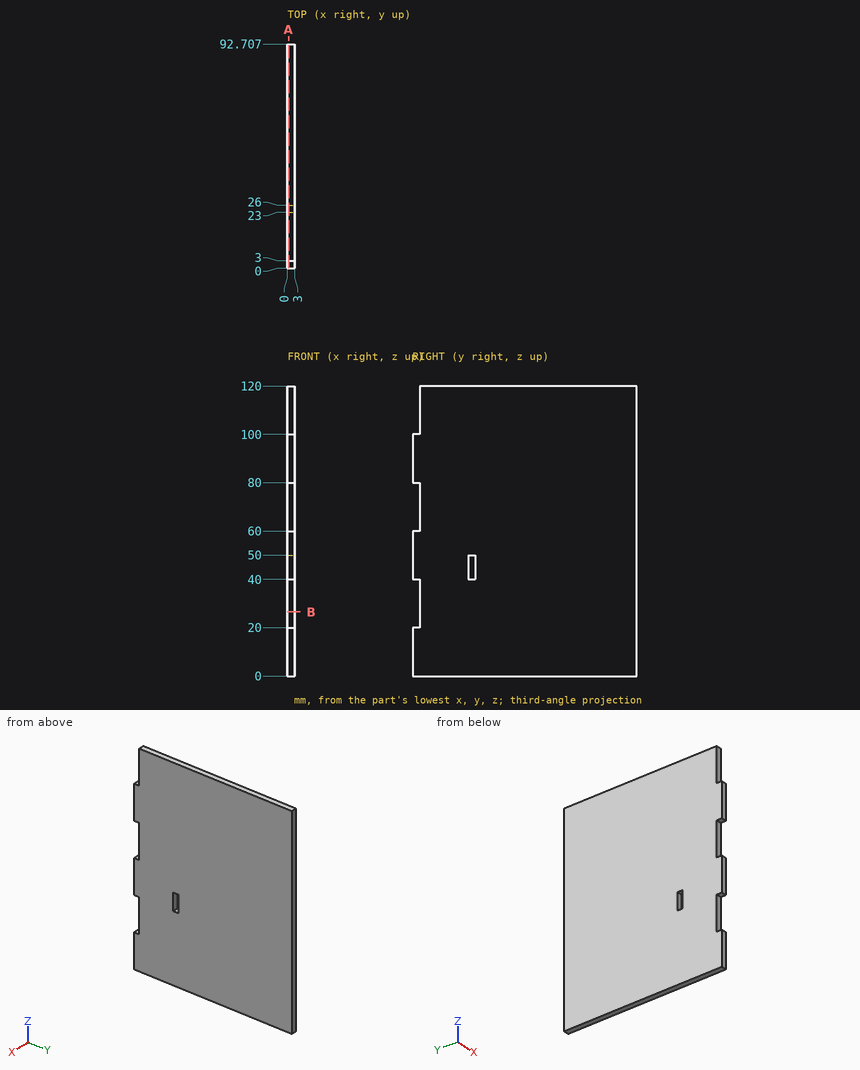
Drawing for the job (mm, zero at the part's lowest x, y, z). Round coordinates to 2 decimals unless told otherwise and drop trailing zeros. Write each loop counter-clockwise with the first axis right and the second up, starting at its lowest first coordinate (ties: lowest second). Pieces come first, ordered by that corner, then holes. Notation, with made-up numbers: M 6.25,15.5 L 17.25,15.5 A25 cw 17.25,28.5 Z; hole C 37,2 d3. An arc over 180 degrees is marked long. Answer in a Markdown table with one row per item.
1. Saw through at B-B (z = 26.5). List the corners of the cut face in (x, y), and give its area (3 significant figures).
Geometry check:
| item | result |
|---|---|
| outline | M 0,3 L 3,3 L 3,92.71 L 0,92.71 Z |
| area | 269 mm2 |
2. Flat gauge pin, fed straight in: P1, Ø0.9, axis at x = 2, z = 108.5, coming from the -Y side. Where does the tip first touch, or does it go through?
Geometry check:
| item | result |
|---|---|
| P1 | y = 3 |
3. Saw through at A-A (x = 0.5). List the corners of the cut face in (y, z), and give its area (3 significant figures).
Geometry check:
| item | result |
|---|---|
| outline | M 0,0 L 92.71,0 L 92.71,120 L 3,120 L 3,100 L 0,100 L 0,80 L 3,80 L 3,60 L 0,60 L 0,40 L 3,40 L 3,20 L 0,20 Z; hole M 23,40 L 26,40 L 26,50 L 23,50 Z |
| area | 10,900 mm2 |
4. Probe L1, parallel to Z at x = 2.8, y = 24; L2, parallel to Y at x = 1.05, z = 70; L3, parallel to Y at x = 0.75, z = 41. List the from-to ranges inside material, lowest first. Write a range as [from, to].
Geometry check:
| item | result |
|---|---|
| L1 | [0, 40], [50, 120] |
| L2 | [3, 92.71] |
| L3 | [0, 23], [26, 92.71] |
